Source: CAD feature listing. Evaluate the final solid. Frame: model axes, mm. A direction names the side the tool comes from. Give positions to 0.01 mm unless a question says otherwise; leave off trailing zeros. Order: outer loops, then holes, each group sorted by start corner. A loop starts at its lowest first (then second) coordinate and runs counter-clockwise, first axis right, second up. Notation, with made-up numbers: M 50.25,45 L 94.25,45 A15 cw 94.25,57 Z; hole C 33.25,-4.5 d8. An arc over 180 degrees is marked long. Answer as a JSON object with one key per item and string values. Group by question number.
1. Section query A-A (y = 5.5). Output: boundary loops of the cut face in (x, z).
2. Set-up query: faces 1 (the flat face through (0, 0, 0)), 2 (the flat face through (-14.5, 7.737, 0)). Return all of +Z, -Z, +X, -X, +Y, -Y with unobstructed straight access to the full face (end or side cutting, diameter ignored); none if empty.
3. Material intervals for L1, parallel to X at y = 5.75, z = 0.35; L2, parallel to Y at x = -4.5, z = 2; L3, parallel to Y at x = 13.75, z = 1.15, sorted ascending. Write a range as [from, to].
4. Section query B-B (z = -0.75). Output: boundary loops of the cut face in (x, y), plus the area to 3 significant figures.
5. Pin query (flat end, axial travel): P1, Ø1.5, axis at x = -2.5, z = 0.5, coming from the +Y side; P2, Ø2, axis at x = -6, y = 1.5, coming from the -Z side. Return the tip coordinate at first contact, or that it passes through.
6. Section query C-C (x = 1.25). Output: boundary loops of the cut face in (y, z), plus the area to 3 significant figures.
from build123d import *

# Parameters (mm, degrees)
SKETCH1_W                    = 30
SKETCH1_H                    = 5
BASE_FLANGE1_DEPTH           = 1
EDGE_FLANGE1_STRIP_W         = 5.4732
EDGE_FLANGE1_STRIP_H         = 1
EDGE_FLANGE1_STRIP_CUT_DEPTH = 5
EDGE_FLANGE1_DEPTH           = 5
EDGE_FLANGE2_STRIP_W         = 5.4732
EDGE_FLANGE2_STRIP_H         = 1
EDGE_FLANGE2_STRIP_CUT_DEPTH = 5
EDGE_FLANGE2_DEPTH           = 5


# Sheet-metal steps are written as plain solids
with BuildPart() as part:
    # Sketch1 → Base-Flange1 (new body)
    with BuildSketch(Plane(origin=(0, 0, 0), x_dir=(1, 0, 0), z_dir=(0, 1, 0))):
        Rectangle(SKETCH1_W, SKETCH1_H)
    extrude(amount=-BASE_FLANGE1_DEPTH)

    # Edge-Flange1 strip (across the edge) → Edge-Flange1 strip cut (cut)
    with BuildSketch(Plane(origin=(-15, 0, -2.5), x_dir=(1, 0, 0), z_dir=(0, 0, 1))):
        with Locations((-1, -0.5)):
            Rectangle(EDGE_FLANGE1_STRIP_W, EDGE_FLANGE1_STRIP_H)
    extrude(amount=EDGE_FLANGE1_STRIP_CUT_DEPTH, mode=Mode.SUBTRACT)

    # Edge-Flange1 section (across the edge) → Edge-Flange1 (add)
    with BuildSketch(Plane(origin=(-15, 0, -2.5), x_dir=(1, 0, 0), z_dir=(0, 0, 1))):
        with BuildLine():
            Line((0, 0.7366), (0, 7.7366))
            Line((0, 7.7366), (1, 7.7366))
            Line((1, 7.7366), (1, 0.7366))
            ThreePointArc((1, 0.7366), (1.215745145, 0.215745145), (1.7366, 0))
            Line((1.7366, 0), (1.7366, -1))
            ThreePointArc((1.7366, -1), (0.508638364, -0.491361636), (0, 0.7366))
        make_face()
    extrude(amount=EDGE_FLANGE1_DEPTH)

    # Edge-Flange2 strip (across the edge) → Edge-Flange2 strip cut (cut)
    with BuildSketch(Plane(origin=(15, 0, 2.5), x_dir=(-1, 0, 0), z_dir=(0, 0, -1))):
        with Locations((-1, -0.5)):
            Rectangle(EDGE_FLANGE2_STRIP_W, EDGE_FLANGE2_STRIP_H)
    extrude(amount=EDGE_FLANGE2_STRIP_CUT_DEPTH, mode=Mode.SUBTRACT)

    # Edge-Flange2 section (across the edge) → Edge-Flange2 (add)
    with BuildSketch(Plane(origin=(15, 0, 2.5), x_dir=(-1, 0, 0), z_dir=(0, 0, -1))):
        with BuildLine():
            Line((0, 0.7366), (0, 7.7366))
            Line((0, 7.7366), (1, 7.7366))
            Line((1, 7.7366), (1, 0.7366))
            ThreePointArc((1, 0.7366), (1.215745145, 0.215745145), (1.7366, 0))
            Line((1.7366, 0), (1.7366, -1))
            ThreePointArc((1.7366, -1), (0.508638364, -0.491361636), (0, 0.7366))
        make_face()
    extrude(amount=EDGE_FLANGE2_DEPTH)


solid = part.part
Answer sheet:
{
 "1": {"outline": "M -15,-2.5 L -14,-2.5 L -14,2.5 L -15,2.5 Z; M 14,-2.5 L 15,-2.5 L 15,2.5 L 14,2.5 Z"},
 "2": {"face 1": "+Z, -Z, +Y", "face 2": "+Z, -Z, +X, -X, +Y"},
 "3": {"L1": "[-15, -14], [14, 15]", "L2": "[-1, 0]", "L3": "[-0.93, 0.18]"},
 "4": {"outline": "M -15,0.74 A1.74 ccw -13.26,-1 L 13.26,-1 A1.74 ccw 15,0.74 L 15,7.74 L 14,7.74 L 14,0.74 A0.74 cw 13.26,0 L -13.26,0 A0.74 cw -14,0.74 L -14,7.74 L -15,7.74 Z", "area": "44.4 mm^2"},
 "5": {"P1": "y = 0", "P2": "through"},
 "6": {"outline": "M -1,-2.5 L 0,-2.5 L 0,2.5 L -1,2.5 Z", "area": "5.00 mm^2"}
}
